Drawing for the job (mm, zero at the part's lowest x, y, z). A direction names the side the tool comes from. Coordinates: 2 decimals unless noted, no trailing zeros. Order: outer loops, then holes, each group sorted by start corner. A loop starts at its lowest first (then second) coordinate and runs counter-clockwise, first axis right, second up. Notation, with made-up numbers: (-29.5, 80) -> (-2.5, 80) arc R10 ccw to (-2.5, 93) -> close; hole circle Ø1 at (66, 37). An arc over 180 degrees is marked (long way). Write each question's results on one line, items separated by ' | '.
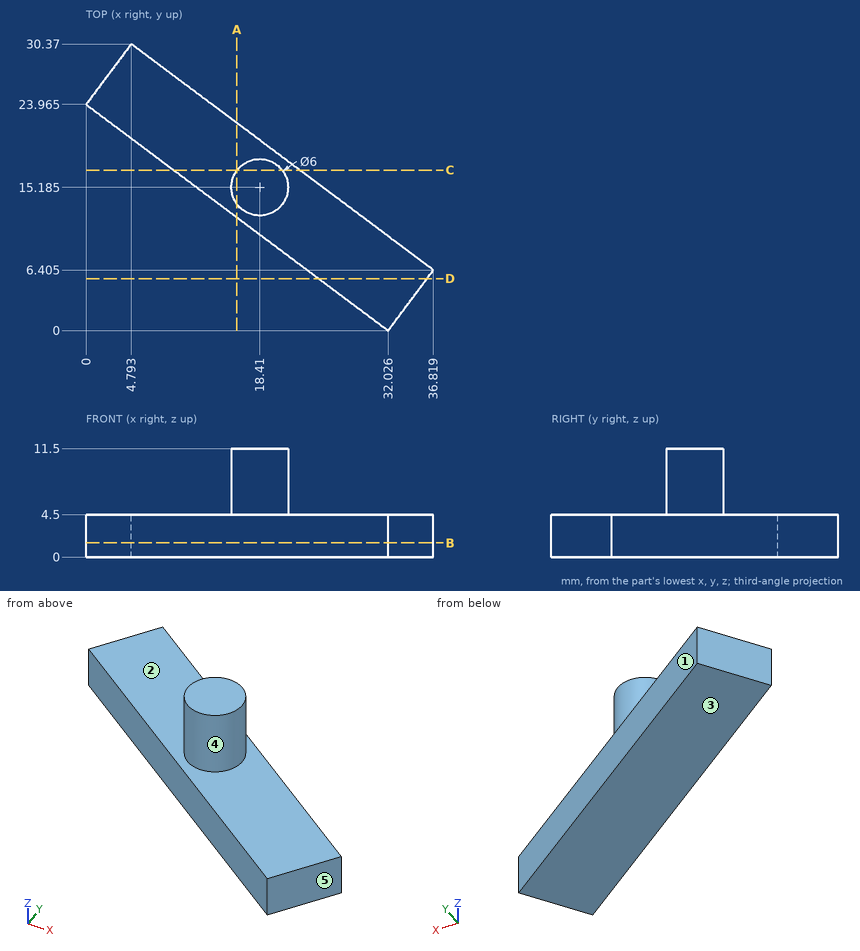
Item 1: Slice it at B-B, the plane z = 1.5. List the corners of the cut face in (x, y) (1 decimal), and give its area (3 significant figures).
Answer:
outline: (0, 24) -> (32, 0) -> (36.8, 6.4) -> (4.8, 30.4) -> close | area: 320 mm^2
Item 2: Slice it at C-C, the plane y = 17. List the corners of the cut face in (x, z).
Answer:
outline: (9.31, 0) -> (22.66, 0) -> (22.66, 4.5) -> (20.8, 4.5) -> (20.8, 11.5) -> (16.02, 11.5) -> (16.02, 4.5) -> (9.31, 4.5) -> close
Item 3: Tool access for the marked faces 4 and 5: list every direction of +Z, -Z, +X, -X, +Y, -Y with a clear straight run to the whole face (end or side of a thin tool).
Answer:
face 4: +Z | face 5: +Z, -Z, +X, -Y
Item 4: Pin check, flat tips, straight feed: pin 1 (9 mm diameter, centred on x = 11, y = 19.5, fed in from +Z); pin 2 (5 mm diameter, centred on x = 22, z = 2, fed in from +Y) (1 decimal); pin 3 (3 mm diameter, centred on x = 22.5, z = 4.5, fed in from -Y) (1 decimal). Stop position of each tip, or through.
Answer:
pin 1: stops at z = 4.5 | pin 2: stops at y = 19.4 | pin 3: stops at y = 6
Item 5: Drill centre lines: line 1 (Z direction, x = 22, y = 15); line 2 (X direction, y = 2, z = 3.5) (1 decimal); line 3 (Y direction, x = 30, z = 3.5) (1 decimal). Where is each one in solid material? Low to high. Write a range as from..to.
Answer:
line 1: z = 0..4.5 | line 2: x = 29.4..33.5 | line 3: y = 1.5..11.5
Item 6: Slice it at D-D, the plane y = 5.5. List the corners of the cut face in (x, z), and give its area (3 significant figures).
Answer:
outline: (24.68, 0) -> (36.14, 0) -> (36.14, 4.5) -> (24.68, 4.5) -> close | area: 51.6 mm^2
Item 7: Slice it at A-A, the plane x = 16. List the corners of the cut face in (y, z).
Answer:
outline: (11.99, 0) -> (21.98, 0) -> (21.98, 4.5) -> (16.97, 4.5) -> (16.97, 11.5) -> (13.4, 11.5) -> (13.4, 4.5) -> (11.99, 4.5) -> close
Item 8: Pull direction Z, two halves, no side cores. Call the marked faces 1, 2 and 3: released by +Z, released by -Z, zero draft, split by the parting line, or undercut.
Answer:
face 1: zero draft | face 2: released by +Z | face 3: released by -Z
